Verification items for the finished model (mm, model axes). Face numbers are marked on the shaded views. A direction names the side the tool comes from. Round coordinates to 2 decimals unless told otherwise and drop trailing zeros. Order: outer loops, then holes, each group sorted by start corner. A loop starts at its lowest first (then second) coordinate and runs counter-clockwise, first axis right, second up. Notation, with made-up numbers: (60, 40.5) -> (82, 40.5) arc R14 ccw to (82, 54.5) -> close; hole circle Ø8 at (72.25, -18.5). An arc over 180 degrees is marked (long way). Put each result on its own line as item: value.
```python
from build123d import *

# Parameters (mm, degrees)
SKETCH1_R           = 5
BOSS_EXTRUDE1_DEPTH = 5
CHAMFER1_SIZE       = 0.5
SKETCH2_R           = 7
SKETCH2_R_2         = 5
BOSS_EXTRUDE2_DEPTH = 10
BOSS_EXTRUDE2_DRAFT = 3


with BuildPart() as part:
    # Sketch1 → Boss-Extrude1 (new body)
    with BuildSketch(Plane(origin=(0, 0, 0), x_dir=(1, 0, 0), z_dir=(0, 1, 0))):
        Polygon((7.08862867, -10.539671575), (12.671937667, 0.869096719), (5.583308997, 11.408768294), (-7.08862867, 10.539671575), (-12.671937667, -0.869096719), (-5.583308997, -11.408768294), align=None)
        with Locations(Location((0, 0, 0), (0, 0, 270))):
            Circle(SKETCH1_R, mode=Mode.SUBTRACT)
    extrude(amount=BOSS_EXTRUDE1_DEPTH)

    # Chamfer1
    chamfer1_edges = [part.edges().sort_by_distance(p)[0] for p in [
        (9.127623332, 5, -6.138932506),
        (-0.752659837, 5, -10.974219934),
        (-9.880283168, 5, -4.835287428),
        (-9.127623332, 5, 6.138932506),
        (0.752659837, 5, 10.974219934),
        (9.880283168, 5, 4.835287428),
    ]]
    chamfer(chamfer1_edges, length=CHAMFER1_SIZE)


with BuildPart() as boss_extrude2_tool:
    # Sketch2 → Boss-Extrude2 (with draft: the straight prism first)
    with BuildSketch(Plane(origin=(0, 5, 0), x_dir=(1, 0, 0), z_dir=(0, 1, 0))):
        Circle(SKETCH2_R)
        with Locations(Location((0, 0, 0), (0, 0, 270))):
            Circle(SKETCH2_R_2, mode=Mode.SUBTRACT)
    extrude(amount=BOSS_EXTRUDE2_DEPTH)
    # Boss-Extrude2: the draft: its side faces are tilted about the plane it starts from
    boss_extrude2_sides = [boss_extrude2_tool.faces().sort_by_distance(p)[0] for p in [
        (-7, 10, 0),
        (0, 10, -5),
    ]]
    draft(boss_extrude2_sides, Plane(origin=(0, 5, 0), x_dir=(1, 0, 0), z_dir=(0, 1, 0)), BOSS_EXTRUDE2_DRAFT)


with BuildPart() as part_1:
    add(part.part)

    # Boss-Extrude2: add boss_extrude2_tool
    add(boss_extrude2_tool.part)


solid = part_1.part
```
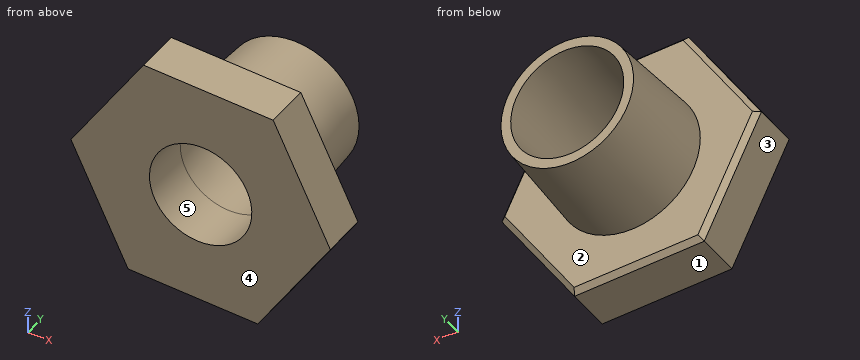
Item 1: Sectioned sample at A-A, the plane y = 3.5. Record the boundary of the cut face in (x, z), then the cut area to 3 significant figures.
Geometry check:
outline: (-12.67, 0.87) -> (-7.09, -10.54) -> (5.58, -11.41) -> (12.67, -0.87) -> (7.09, 10.54) -> (-5.58, 11.41) -> close; hole circle Ø10 at (0, 0)
area: 341 mm2
Item 2: Sectioned sample at D-D, the plane z = 7.5. Record the boundary of the cut face in (x, y), then the cut area to 3 significant figures.
Geometry check:
outline: (-8.21, 0) -> (8.58, 0) -> (8.58, 4.5) -> (8.02, 5) -> (-7.61, 5) -> (-8.21, 4.5) -> close
area: 83.7 mm2
Item 3: Tool access check on the marked faces 1 and 2. Record the directions out of +Z, -Z, +X, -X, +Y, -Y that give a thin tool (end or side, any length) a straight path to the whole face; none if there is none.
Geometry check:
face 1: -Z, -X, +Y, -Y
face 2: +Y
Item 4: Sectioned sample at C-C, the plane z = 0. Record the boundary of the cut face in (x, y).
Geometry check:
outline: (-12.25, 0) -> (-5, 0) -> (-5, 5) -> (-5.52, 15) -> (-6.48, 15) -> (-7, 5) -> (-11.69, 5) -> (-12.25, 4.5) -> close; (5, 0) -> (12.25, 0) -> (12.25, 4.5) -> (11.69, 5) -> (7, 5) -> (6.48, 15) -> (5.52, 15) -> (5, 5) -> close
Item 5: Material ranges on line 1 along Y through (x, z) = (-2.5, -8.5); line 2 along X through (y, z) = (3.9, 0); line 3 along X through (y, z) = (11, 2), recorded low to high.
Geometry check:
line 1: 0 to 5
line 2: -12.25 to -5, 5 to 12.25
line 3: -6.38 to -4.92, 4.92 to 6.38
Item 6: Release check for a two-part mould opening along Z. For the marked faces 3, 4 and 5 record: pulls with the +Z half, pulls with the -Z half, needs draft (parallel to the pull), parting line crosses it, or undercut.
Geometry check:
face 3: pulls with the -Z half
face 4: needs draft
face 5: undercut
Item 7: Sectioned sample at B-B, the plane x = 0. Record the boundary of the cut face in (y, z).
Geometry check:
outline: (0, -11.03) -> (4.5, -11.03) -> (5, -10.52) -> (5, -7) -> (15, -6.48) -> (15, -5.52) -> (5, -5) -> (0, -5) -> close; (0, 5) -> (5, 5) -> (15, 5.52) -> (15, 6.48) -> (5, 7) -> (5, 10.52) -> (4.5, 11.03) -> (0, 11.03) -> close
Item 8: Depth check by flat-ended pin: pin 1 Ø6 at (y, z) = (12, 5.5) entering from -X; pin 2 Ø5 at (x, y) = (7, 2.5) entering from +Z; pin 3 Ø3 at (x, z) = (-4.5, 8) entering from +Y. Enter the tip coordinate at first touch or a pass-through.
Geometry check:
pin 1: x = -6.16
pin 2: z = 10.72
pin 3: y = 5
